Source: three-view drawing plus pictorial views. Frame: mm from the lowest corner of the part. Give positions to 0.01 mm unless a question says otherwise; leave off trailing zeros. Loops run counter-clockwise (first coordinate to the right, second up) from the corner with the lowest first, then second, coordinate; pieces in that order, holes last. Notation, with made-up numbers: (10, 39.5) - (22, 39.5) arc R18 cw to (22, 48.5) - close; hole circle Ø6 at (-27, 55). An arc over 180 degrees is marked (long way). Put each result on its own line as item: value.
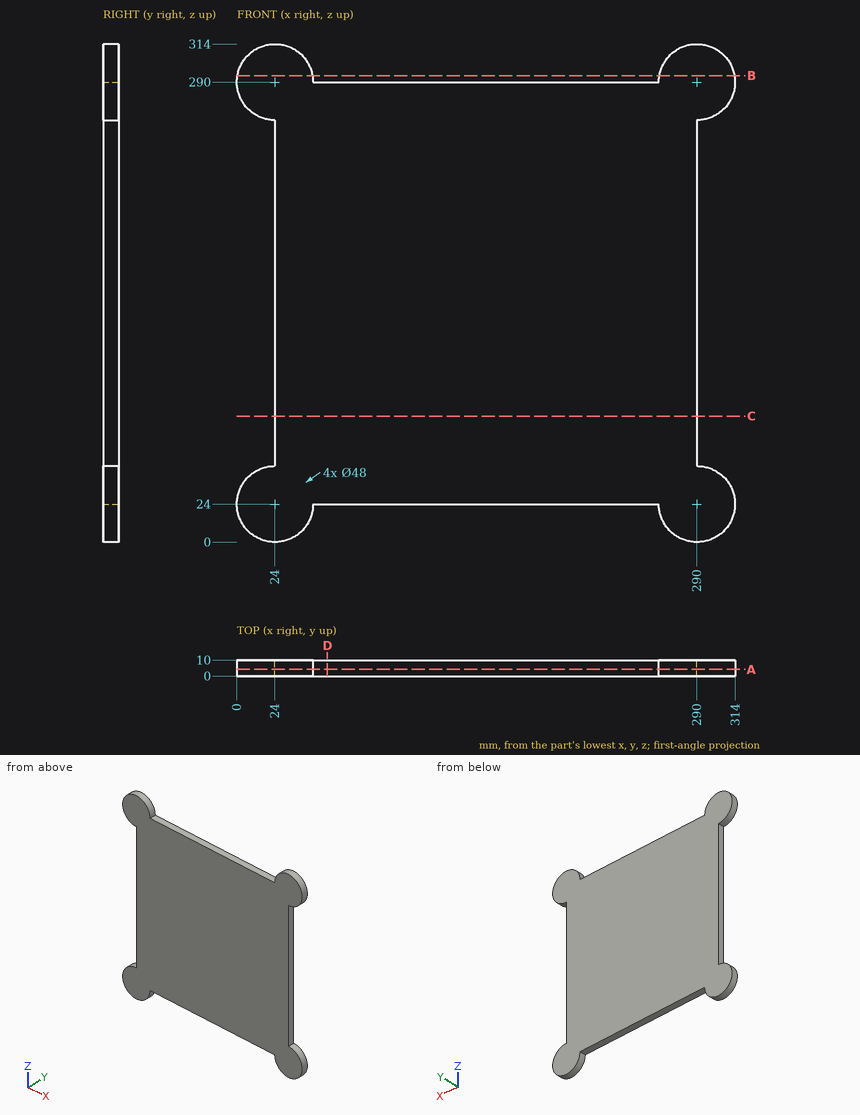
1) Pin query (flat end, axial travel): P1, Ø1, axis at x = 229.5, y = 4, coming from the +Z side; P2, Ø3, axis at y = 7, z = 185, coming from the -X side; P3, Ø1.5, axis at x = 31.5, y = 9, coming from the +Z side. Return the tip coordinate at first contact, or that it passes through.
Check result:
P1: z = 290
P2: x = 24
P3: z = 313.03
2) Section query B-B, the plane z = 294. Output: boundary loops of the cut face in (x, y), plus the area to 3 significant figures.
Check result:
outline: (0.34, 0) - (47.66, 0) - (47.66, 10) - (0.34, 10) - close; (266.34, 0) - (313.66, 0) - (313.66, 10) - (266.34, 10) - close
area: 947 mm²
3) Material intervals for line 1 along Z through (x, y) = (94, 6.5); line 2 along X through (y, z) = (4.25, 270.5), sorted ascending. Write a range as [from, to].
Check result:
line 1: [24, 290]
line 2: [10.01, 303.99]
4) Section query C-C, the plane z = 79.5. Output: boundary loops of the cut face in (x, y).
Check result:
outline: (24, 0) - (290, 0) - (290, 10) - (24, 10) - close
5) Section query D-D, the plane x = 57. Output: boundary loops of the cut face in (y, z).
Check result:
outline: (0, 24) - (10, 24) - (10, 290) - (0, 290) - close
6) Section query A-A, the plane y = 4.25. Output: boundary loops of the cut face in (x, z).
Check result:
outline: (24, 48) arc R24 ccw (long way) to (48, 24) - (266, 24) arc R24 ccw (long way) to (290, 48) - (290, 266) arc R24 ccw (long way) to (266, 290) - (48, 290) arc R24 ccw (long way) to (24, 266) - close
